Can you work these out from the model? Positions are in its coordinate system, mm. A direction names the side the tool comes from. Coordinates: 2 decimals unless noted, no trailing zeros. Loops run counter-clockwise (first coordinate to the right, second up) from the corner with the lowest first, then second, coordinate; pieces in that order, holes last.
```python
from build123d import *

# Parameters (mm, degrees)
SKETCH1_W           = 23
SKETCH1_H           = 65
BOSS_EXTRUDE1_DEPTH = 66
SKETCH2_W           = 60
SKETCH2_H           = 17
CUT_EXTRUDE1_DEPTH  = 66
CUT_EXTRUDE2_REACH  = 25
SKETCH3_W           = 32
SKETCH3_H           = 65
CUT_EXTRUDE3_REACH  = 25
SKETCH5_R           = 2
SKETCH6_W           = 17
SKETCH6_H           = 15
CUT_EXTRUDE4_DEPTH  = 20


with BuildPart() as part:
    # Sketch1 → Boss-Extrude1 (new body)
    with BuildSketch(Plane(origin=(0, 0, 0), x_dir=(0, 0, -1), z_dir=(1, 0, 0))):
        with Locations((-11.5, -32.5)):
            Rectangle(SKETCH1_W, SKETCH1_H)
    extrude(amount=-BOSS_EXTRUDE1_DEPTH)

    # Sketch2 → Cut-Extrude1 (cut, through all)
    with BuildSketch(Plane(origin=(0, 0, 0), x_dir=(1, 0, 0), z_dir=(0, 1, 0))):
        with Locations((-33, -11.5)):
            Rectangle(SKETCH2_W, SKETCH2_H)
    extrude(amount=-CUT_EXTRUDE1_DEPTH, mode=Mode.SUBTRACT)

    # Sketch3 → Cut-Extrude2 (cut, up to next)
    with BuildSketch(Plane.XY.offset(23), mode=Mode.PRIVATE) as cut_extrude2_sk1:
        with Locations((-33, -32.5)):
            Rectangle(SKETCH3_W, SKETCH3_H)
    cut_extrude2_tool1 = extrude(cut_extrude2_sk1.sketch, amount=-CUT_EXTRUDE2_REACH, mode=Mode.PRIVATE) & part.part
    add(cut_extrude2_tool1.solids().sort_by_distance((-33, -32.5, 23))[0], mode=Mode.SUBTRACT)

    # Sketch5 → Cut-Extrude3 (cut, up to next)
    with BuildSketch(Plane(origin=(0, 0, 0), x_dir=(-1, 0, 0), z_dir=(0, 0, -1)), mode=Mode.PRIVATE) as cut_extrude3_sk1:
        with Locations((8, -7)):
            Circle(SKETCH5_R)
    cut_extrude3_tool1 = extrude(cut_extrude3_sk1.sketch, amount=-CUT_EXTRUDE3_REACH, mode=Mode.PRIVATE) & part.part
    add(cut_extrude3_tool1.solids().sort_by_distance((-8, -7, 0))[0], mode=Mode.SUBTRACT)
    # Sketch5 → Cut-Extrude3 (cut, up to next)
    with BuildSketch(Plane(origin=(0, 0, 0), x_dir=(-1, 0, 0), z_dir=(0, 0, -1)), mode=Mode.PRIVATE) as cut_extrude3_sk2:
        with Locations((58, -7)):
            Circle(SKETCH5_R)
    cut_extrude3_tool2 = extrude(cut_extrude3_sk2.sketch, amount=-CUT_EXTRUDE3_REACH, mode=Mode.PRIVATE) & part.part
    add(cut_extrude3_tool2.solids().sort_by_distance((-58, -7, 0))[0], mode=Mode.SUBTRACT)
    # Sketch5 → Cut-Extrude3 (cut, up to next)
    with BuildSketch(Plane(origin=(0, 0, 0), x_dir=(-1, 0, 0), z_dir=(0, 0, -1)), mode=Mode.PRIVATE) as cut_extrude3_sk3:
        with Locations((8, -60)):
            Circle(SKETCH5_R)
    cut_extrude3_tool3 = extrude(cut_extrude3_sk3.sketch, amount=-CUT_EXTRUDE3_REACH, mode=Mode.PRIVATE) & part.part
    add(cut_extrude3_tool3.solids().sort_by_distance((-8, -60, 0))[0], mode=Mode.SUBTRACT)
    # Sketch5 → Cut-Extrude3 (cut, up to next)
    with BuildSketch(Plane(origin=(0, 0, 0), x_dir=(-1, 0, 0), z_dir=(0, 0, -1)), mode=Mode.PRIVATE) as cut_extrude3_sk4:
        with Locations((58, -60)):
            Circle(SKETCH5_R)
    cut_extrude3_tool4 = extrude(cut_extrude3_sk4.sketch, amount=-CUT_EXTRUDE3_REACH, mode=Mode.PRIVATE) & part.part
    add(cut_extrude3_tool4.solids().sort_by_distance((-58, -60, 0))[0], mode=Mode.SUBTRACT)
    # Sketch5 → Cut-Extrude3 (cut, up to next)
    with BuildSketch(Plane(origin=(0, 0, 0), x_dir=(-1, 0, 0), z_dir=(0, 0, -1)), mode=Mode.PRIVATE) as cut_extrude3_sk5:
        with BuildLine():
            Line((38, -37.5), (38, -42.5))
            ThreePointArc((38, -42.5), (33, -47.5), (28, -42.5))
            Line((28, -42.5), (28, -37.5))
            ThreePointArc((28, -37.5), (33, -32.5), (38, -37.5))
        make_face()
    cut_extrude3_tool5 = extrude(cut_extrude3_sk5.sketch, amount=-CUT_EXTRUDE3_REACH, mode=Mode.PRIVATE) & part.part
    add(cut_extrude3_tool5.solids().sort_by_distance((-33, -40, 0))[0], mode=Mode.SUBTRACT)
    # Sketch5 → Cut-Extrude3 (cut, up to next)
    with BuildSketch(Plane(origin=(0, 0, 0), x_dir=(-1, 0, 0), z_dir=(0, 0, -1)), mode=Mode.PRIVATE) as cut_extrude3_sk6:
        with BuildLine():
            Line((17, -37.5), (17, -42.5))
            ThreePointArc((17, -42.5), (15, -44.5), (13, -42.5))
            Line((13, -42.5), (13, -37.5))
            ThreePointArc((13, -37.5), (15, -35.5), (17, -37.5))
        make_face()
    cut_extrude3_tool6 = extrude(cut_extrude3_sk6.sketch, amount=-CUT_EXTRUDE3_REACH, mode=Mode.PRIVATE) & part.part
    add(cut_extrude3_tool6.solids().sort_by_distance((-15, -40, 0))[0], mode=Mode.SUBTRACT)
    # Sketch5 → Cut-Extrude3 (cut, up to next)
    with BuildSketch(Plane(origin=(0, 0, 0), x_dir=(-1, 0, 0), z_dir=(0, 0, -1)), mode=Mode.PRIVATE) as cut_extrude3_sk7:
        with BuildLine():
            Line((53, -37.5), (53, -42.5))
            ThreePointArc((53, -42.5), (51, -44.5), (49, -42.5))
            Line((49, -42.5), (49, -37.5))
            ThreePointArc((49, -37.5), (51, -35.5), (53, -37.5))
        make_face()
    cut_extrude3_tool7 = extrude(cut_extrude3_sk7.sketch, amount=-CUT_EXTRUDE3_REACH, mode=Mode.PRIVATE) & part.part
    add(cut_extrude3_tool7.solids().sort_by_distance((-51, -40, 0))[0], mode=Mode.SUBTRACT)

    # Sketch6 → Cut-Extrude4 (cut)
    with BuildSketch(Plane.XY.offset(23)):
        with Locations((-57.5, -7.5)):
            Rectangle(SKETCH6_W, SKETCH6_H)
        with Locations((-8.5, -7.5)):
            Rectangle(SKETCH6_W, SKETCH6_H)
    extrude(amount=-CUT_EXTRUDE4_DEPTH, mode=Mode.SUBTRACT)


solid = part.part
```
(1) If we mould it in two halves opening along Z, with no side actions, what happens to faces 1 (the flat face through (-63, -40, 12)), 2 (the flat face through (-28, -40, 1)), 3 (the flat face through (-57, -40, 23))? For each: released by +Z, released by -Z, zero draft, split by the parting line, or undercut.
Check values:
face 1: undercut
face 2: zero draft
face 3: released by +Z
(2) I want a section at D-D on z = 2. Write out the boundary of the cut face in (x, y).
Check values:
outline: (-66, -65) - (0, -65) - (0, 0) - (-66, 0) - close; hole circle Ø4 at (-58, -60); hole circle Ø4 at (-58, -7); hole (-53, -42.5) arc R2 ccw to (-49, -42.5) - (-49, -37.5) arc R2 ccw to (-53, -37.5) - close; hole (-38, -42.5) arc R5 ccw to (-28, -42.5) - (-28, -37.5) arc R5 ccw to (-38, -37.5) - close; hole (-17, -42.5) arc R2 ccw to (-13, -42.5) - (-13, -37.5) arc R2 ccw to (-17, -37.5) - close; hole circle Ø4 at (-8, -60); hole circle Ø4 at (-8, -7)
(3) I'm going to push flat-ended pins straight in: pin 1 (3 mm diameter, centred on y = -28, z = 4.5, fed in from +X); pin 2 (2 mm diameter, centred on x = -59, z = 5, fed in from +Y); pin 3 (5 mm diameter, centred on x = -18, y = -11, fed in from +Z); pin 4 (13.5 mm diameter, centred on x = -60.5, z = 10.5, fed in from +Y). Where does each tip first touch, or does it pass through?
Check values:
pin 1: stops at x = 0
pin 2: passes through
pin 3: stops at z = 3
pin 4: stops at y = -15
(4) I want a section at C-C on x = -33. Write out the boundary of the cut face in (y, z), then the cut area to 3 significant figures.
Check values:
outline: (-65, 0) - (-47.5, 0) - (-47.5, 3) - (-65, 3) - close; (-32.5, 0) - (0, 0) - (0, 3) - (-32.5, 3) - close
area: 150 mm2
(5) If I drill on probe 1 along Y at (x, z) = (-58, 1); probe 2 along X at (y, z) = (-23.5, 10.75); probe 3 along Z at (x, y) = (-5, -48), over which ranges is the centre line in solid material (lowest first)?
Check values:
probe 1: y = -65 to -62, -58 to -9, -5 to 0
probe 2: x = -66 to -63, -3 to 0
probe 3: z = 0 to 3, 20 to 23
(6) I want a section at B-B on y = -39. Write out the boundary of the cut face in (x, z).
Check values:
outline: (-66, 0) - (-53, 0) - (-53, 3) - (-63, 3) - (-63, 20) - (-49, 20) - (-49, 23) - (-66, 23) - close; (-49, 0) - (-38, 0) - (-38, 3) - (-49, 3) - close; (-28, 0) - (-17, 0) - (-17, 3) - (-28, 3) - close; (-17, 20) - (-3, 20) - (-3, 3) - (-13, 3) - (-13, 0) - (0, 0) - (0, 23) - (-17, 23) - close
(7) Which directions (+Z, -Z, +X, -X, +Y, -Y) give clear straight access to the entire face, cutting with the end or side of a thin tool? Please do faces 4 (the flat face through (-49, -40, 22)), 5 (the cylindrical face through (-32.9, -32.5, 1.5)), 6 (the cylindrical face through (-15, -35.5, 1.5)).
Check values:
face 4: +Z, +Y, -Y
face 5: +Z, -Z
face 6: -Z
(8) I want a section at A-A on z = 15.25. Write out the boundary of the cut face in (x, y).
Check values:
outline: (-66, -65) - (-63, -65) - (-63, -15) - (-66, -15) - close; (-3, -65) - (0, -65) - (0, -15) - (-3, -15) - close
